Part model, mm, in its own coordinate system. A direction names the side the tool comes from. Round coordinates to 2 decimals unless told otherwise and drop trailing zeros. Loops run counter-clockwise (first coordinate to the right, second up) from the corner with the lowest first, then second, coordinate; pieces in that order, holes last.
(1) Cut at C-C on z = 33. List the corners of the cut face in (x, y).
(2) Cut at B-B on x = 23.5. List the corners of the cut face in (y, z), then the cut area to 3 significant figures.
(3) Flat gauge pins, fed straight in: pin 1 (3.5 mm diameter, centred on y = 0, z = 33, fed in from +X); pin 2 (3 mm diameter, centred on x = 3.62, z = -1, fed in from +Y); pin 3 (10 mm diameter, centred on y = -15.5, z = 23.5, fed in from +X). Where does each tip first touch, or does it go through?
(4) Cut at A-A on y = 0. List the corners of the cut face in (x, z).
(5) Probe probe 1 along Y at (x, z) = (16.5, 0); probe 2 along Y at (x, z) = (1, 0); probe 3 along X at (y, z) = (31, -1). List the from-to ranges inside material, lowest first.
(6) Cut at D-D on z = -1. List the corners of the cut face in (x, y), then the cut area to 3 significant figures.
(7) Tool access for faces 1 (the face through (15, 0, -35.36)), 2 (the face through (3.7, 31.74, -2.75)), 3 (the face through (15, 35.36, 0)), 4 (the face through (32.96, -0.9, 2.86)), 5 (the face through (3, 0, -3)): list every direction of +Z, -Z, +X, -X, +Y, -Y with a clear straight run to the whole face (end or side of a thin tool).
(8) Mould opens along Z. For faces 6 (the face through (15.21, 33.601, 1.908)), 7 (the face through (4, 29.36, -1)), 8 (the face through (15.21, 32.51, -32.35)), 9 (the face through (15, -35.36, 0)) say: +Z half, -Z half, draft (parallel to the pull), parting line (faces both ways), or undercut.
from build123d import *

# Parameters (mm, degrees)
SKETCH_1_W               = 70.72
SKETCH_1_H               = 70.72
EXTRUDE_1_DEPTH          = 30
SKETCH_2_R               = 3
CUT_EXTRUDE_1_DEPTH      = 6
SKETCH_3_R               = 3
EXTRUDE_2_DEPTH          = 6
SKETCH_5_R               = 1.75
CUT_EXTRUDE_2_DEPTH      = 6
CUT_EXTRUDE_3_DEPTH      = 59.315171268
CUT_EXTRUDE_3_DEPTH_BACK = 59.315171268
SKETCH_7_R               = 2
FILLET_1_R               = 10
FILLET_2_R               = 10
FILLET_3_R               = 10
FILLET_4_R               = 10


with BuildPart() as part:
    # 草图1 → 凸台-拉伸1 (new body)
    with BuildSketch(Plane(origin=(0, 0, 0), x_dir=(0, 0, -1), z_dir=(1, 0, 0))):
        Rectangle(SKETCH_1_W, SKETCH_1_H)
    extrude(amount=EXTRUDE_1_DEPTH)

    # 草图2 → 切除-拉伸1 (cut)
    with BuildSketch(Plane.ZY):
        Circle(SKETCH_2_R)
    extrude(amount=-CUT_EXTRUDE_1_DEPTH, mode=Mode.SUBTRACT)

    # 草图3 → 凸台-拉伸2 (add)
    with BuildSketch(Plane(origin=(30, 0, 0), x_dir=(0, 0, -1), z_dir=(1, 0, 0))):
        with Locations(Location((0, 0, 0), (0, 0, 180))):
            Circle(SKETCH_3_R)
    extrude(amount=EXTRUDE_2_DEPTH)

    # 草图5 → 切除-拉伸2 (cut)
    with BuildSketch(Plane(origin=(0, 35.36, 0), x_dir=(1, 0, 0), z_dir=(0, 1, 0))):
        with Locations(Location((3.62, 1, 0), (0, 0, 270))):
            Circle(SKETCH_5_R)
    extrude(amount=-CUT_EXTRUDE_2_DEPTH, mode=Mode.SUBTRACT)

    # 草图7 → 切除-拉伸3 (cut, two sides: drawn at the far end of the back side and taken through both)
    with BuildSketch(Plane.ZY.offset(-6).offset(-CUT_EXTRUDE_3_DEPTH_BACK)):
        with Locations((0, 33)):
            Circle(SKETCH_7_R)
        with Locations((33, 0)):
            Circle(SKETCH_7_R)
        with Locations((0, -33)):
            Circle(SKETCH_7_R)
        with Locations((-33, 0)):
            Circle(SKETCH_7_R)
    extrude(amount=CUT_EXTRUDE_3_DEPTH + CUT_EXTRUDE_3_DEPTH_BACK, mode=Mode.SUBTRACT)

    # 圆角1
    fillet_1_edges = [part.edges().sort_by_distance(p)[0] for p in [
        (15, 35.36, -35.36),
    ]]
    fillet(fillet_1_edges, radius=FILLET_1_R)

    # 圆角2
    fillet_2_edges = [part.edges().sort_by_distance(p)[0] for p in [
        (15, -35.36, -35.36),
    ]]
    fillet(fillet_2_edges, radius=FILLET_2_R)

    # 圆角3
    fillet_3_edges = [part.edges().sort_by_distance(p)[0] for p in [
        (15, -35.36, 35.36),
    ]]
    fillet(fillet_3_edges, radius=FILLET_3_R)

    # 圆角4
    fillet_4_edges = [part.edges().sort_by_distance(p)[0] for p in [
        (15, 35.36, 35.36),
    ]]
    fillet(fillet_4_edges, radius=FILLET_4_R)


solid = part.part
Final values:
1. outline: (0, -31.81) - (30, -31.81) - (30, -2) - (0, -2) - close; (0, 2) - (30, 2) - (30, 31.81) - (0, 31.81) - close
2. outline: (-35.36, -25.36) arc R10 ccw to (-25.36, -35.36) - (25.36, -35.36) arc R10 ccw to (35.36, -25.36) - (35.36, 25.36) arc R10 ccw to (25.36, 35.36) - (-25.36, 35.36) arc R10 ccw to (-35.36, 25.36) - close; hole circle Ø4 at (-33, 0); hole circle Ø4 at (0, -33); hole circle Ø4 at (0, 33); hole circle Ø4 at (33, 0)
2. area: 4,870 mm2
3. pin 1: passes through
3. pin 2: stops at y = 29.36
3. pin 3: stops at x = 30
4. outline: (0, -35.36) - (30, -35.36) - (30, -35) - (0, -35) - close; (0, -31) - (30, -31) - (30, -3) - (36, -3) - (36, 3) - (30, 3) - (30, 31) - (0, 31) - (0, 3) - (6, 3) - (6, -3) - (0, -3) - close; (0, 35) - (30, 35) - (30, 35.36) - (0, 35.36) - close
5. probe 1: y = -35.36 to -35, -31 to 31, 35 to 35.36
5. probe 2: y = -35.36 to -35, -31 to -3, 3 to 31, 35 to 35.36
5. probe 3: x = 0 to 1.87, 5.37 to 30
6. outline: (0, -35.36) - (30, -35.36) - (30, -34.73) - (0, -34.73) - close; (0, -31.27) - (30, -31.27) - (30, -2.83) - (36, -2.83) - (36, 2.83) - (30, 2.83) - (30, 31.27) - (5.37, 31.27) - (5.37, 29.36) - (1.87, 29.36) - (1.87, 31.27) - (0, 31.27) - (0, 2.83) - (6, 2.83) - (6, -2.83) - (0, -2.83) - close; (0, 34.73) - (1.87, 34.73) - (1.87, 35.36) - (0, 35.36) - close; (5.37, 34.73) - (30, 34.73) - (30, 35.36) - (5.37, 35.36) - close
6. area: 1,900 mm2
7. face 1: -Z, +X, -X, +Y, -Y
7. face 2: +Y
7. face 3: +Z, -Z, +X, -X, +Y
7. face 4: +X
7. face 5: -X
8. face 6: undercut
8. face 7: undercut
8. face 8: -Z half
8. face 9: draft
